Read the model definition and answer for the solid it produces. Units are mm, in the model's axes. A direction names the side the tool comes from. Coordinates: 2 decimals unless noted, no trailing zeros. Write each loop counter-clockwise with the first axis right and the second up, starting at its lowest first coordinate (ties: lowest second). Pieces come first, ordered by that corner, then holes. Notation, with made-up numbers: (21, 22.25) -> (46, 22.25) arc R21 ccw to (46, 46.25) -> close; hole circle Ø8 at (14, 2.5). An arc over 180 degrees is marked (long way). Answer as a JSON object with one key per item and string values. Group by question number.
(1) Which of the six approach directions +Z, -Z, +X, -X, +Y, -Y give full straight-line access (tool end or side, diameter ignored) to faces 4 (the face through (-1, -98, 17)), 5 (the face through (-1.81, -98.95, 15.03)), 6 (the face through (2.028, -105.448, 8.944))?
(2) Find section D-D (x = 4.75). Give the vertices of the cut face in (y, z).
(3) Find section B-B (z = 16.25). Give the vertices of the cut face in (x, y), then the cut area to 3 significant figures.
(4) Find section C-C (x = 2.75). Give the vertices of the cut face in (y, z).
(5) Find section A-A (y = -100.5). Give the vertices of the cut face in (x, z), then the cut area to 3 significant figures.
(6) Straight lines are drawn through the part: L1, parallel to X at y = -101.5, z = 16.5; L2, parallel to Z at x = -3, y = -108.25; L3, parallel to Z at x = 3.25, y = -102.75. For each, find the intervals that lie inside material, in ascending order.
(7) Flat-ended cylindrical pins translate along their axes: P1, Ø6, axis at y = -107, z = 15, coming from the +X side; P2, Ø2.5, axis at x = -1.5, y = -102, coming from the +Z side; P3, Ø1.5, axis at x = 0, z = 12, coming from the -Y side. Find the tip coordinate at first contact, or state that the pin passes through.
(8) For a pull along X with two mould halves and no side action, classify faces 1 (the face through (7, -103, 13)), 2 (the face through (-1.3, -108.59, 9.06)), 3 (the face through (-1.028, -100.284, 8.944)) as +X half, -X half, draft (parallel to the pull), parting line (faces both ways), or undercut.
from build123d import *

# Parameters (mm, degrees)
SKETCH159_R             = 7
PAD068_DEPTH            = 4
SKETCH160_R             = 6
PAD069_DEPTH            = 8
POCKET068_DEPTH         = 20
BODY020_ROLL_ANGLE      = 90
BODY020_PLACEMENT_ANGLE = 30


with BuildPart() as part:
    # Sketch159 → Pad068 (new body)
    with BuildSketch(Plane.XZ):
        Circle(SKETCH159_R)
        Polygon((5.25, 0), (2.625, 4.546633), (-2.625, 4.546633), (-5.25, 0), (-2.625, -4.546633), (2.625, -4.546633), align=None, mode=Mode.SUBTRACT)
    extrude(amount=PAD068_DEPTH)

    # Sketch160 (on Face9 of Pad068) → Pad069 (join)
    with BuildSketch(Plane.XZ.offset(4)):
        Circle(SKETCH160_R)
    extrude(amount=PAD069_DEPTH)

    # Sketch162 (on Face12 of Pad069) → Pocket068 (cut)
    with BuildSketch(Plane.XZ.offset(12)):
        with BuildLine():
            ThreePointArc((2.1, 2.142429), (0, 3), (-2.1, 2.142429))
            Line((-2.1, 2.142429), (-2.1, -2.142429))
            ThreePointArc((-2.1, -2.142429), (0, -3), (2.1, -2.142429))
            Line((2.1, 2.142429), (2.1, -2.142429))
        make_face()
    extrude(amount=-POCKET068_DEPTH, mode=Mode.SUBTRACT)


with BuildPart() as part_1:
    # Body020 roll: moved
    add(part.part.rotate(Axis((0, 0, 0), (1, 0, 0)), BODY020_ROLL_ANGLE))


with BuildPart() as part_2:
    # Body020 placement: moved
    add(part_1.part.moved(Location((0.5, -102.866025, 17))).rotate(Axis((0.5, -102.866025, 17), (0, 0, 1)), BODY020_PLACEMENT_ANGLE))


solid = part_2.part
Results below:
{
 "1": {"face 4": "+Z, +X, -X, +Y, -Y", "face 5": "+Z", "face 6": "+Z, -Z"},
 "2": {"outline": "(-108.43, 13) -> (-107.1, 13) -> (-107.1, 5) -> (-98.63, 5) -> (-98.63, 13) -> (-97.3, 13) -> (-97.3, 17) -> (-100.07, 17) -> (-100.07, 13) -> (-105.66, 13) -> (-105.66, 17) -> (-108.43, 17) -> close"},
 "3": {"outline": "circle Ø14 at (0.5, -102.87); hole (-4.05, -105.49) -> (0.5, -108.12) -> (5.05, -105.49) -> (5.05, -100.24) -> (0.5, -97.62) -> (-4.05, -100.24) -> close", "area": "82.3 mm2"},
 "4": {"outline": "(-109.49, 13) -> (-108.43, 13) -> (-108.43, 5) -> (-104.85, 5) -> (-104.85, 13) -> (-106.82, 13) -> (-106.82, 17) -> (-109.49, 17) -> close; (-102.56, 5) -> (-97.3, 5) -> (-97.3, 13) -> (-96.24, 13) -> (-96.24, 17) -> (-98.92, 17) -> (-98.92, 13) -> (-102.56, 13) -> close"},
 "5": {"outline": "(-6.09, 13) -> (-5.01, 13) -> (-5.01, 5) -> (-1.34, 5) -> (-1.34, 13) -> (-4.05, 13) -> (-4.05, 17) -> (-6.09, 17) -> close; (1.56, 5) -> (6.01, 5) -> (6.01, 13) -> (7.09, 13) -> (7.09, 17) -> (5.05, 17) -> (5.05, 13) -> (1.56, 13) -> close", "area": "81.3 mm2"},
 "6": {"L1": "x = -6.37 to -4.05, 5.05 to 7.37", "L2": "z = 13 to 17", "L3": "z = 5 to 13"},
 "7": {"P1": "stops at x = 7.41", "P2": "stops at z = 13", "P3": "stops at y = -108.87"},
 "8": {"face 1": "draft", "face 2": "parting line", "face 3": "undercut"}
}
